```python
from build123d import *

# Parameters (mm, degrees)
SKETCH1_W                    = 73.025
SKETCH1_H                    = 177.8
BASE_FLANGE1_DEPTH           = 0.508
SKETCH2_W                    = 73.025
SKETCH2_H                    = 6.35
BOSS_EXTRUDE1_DEPTH          = 1.11125
EDGE_FLANGE1_STRIP_W         = 4.2545
EDGE_FLANGE1_STRIP_H         = 0.508
EDGE_FLANGE1_STRIP_CUT_DEPTH = 73.025
EDGE_FLANGE1_DEPTH           = 73.025


# Sheet-metal steps are written as plain solids
with BuildPart() as part:
    # Sketch1 → Base-Flange1 (new body)
    with BuildSketch(Plane(origin=(0, 0, 0), x_dir=(0, 0, -1), z_dir=(1, 0, 0))):
        with Locations((36.5125, 88.9)):
            Rectangle(SKETCH1_W, SKETCH1_H)
    extrude(amount=-BASE_FLANGE1_DEPTH)

    # Sketch2 → Boss-Extrude1 (add)
    with BuildSketch(Plane(origin=(0, 0, 0), x_dir=(0, 0, -1), z_dir=(1, 0, 0))):
        with Locations((36.5125, 174.625)):
            Rectangle(SKETCH2_W, SKETCH2_H)
    extrude(amount=BOSS_EXTRUDE1_DEPTH)

    # Edge-Flange1 strip (across the edge) → Edge-Flange1 strip cut (cut)
    with BuildSketch(Plane(origin=(-0.508, 0, -73.025), x_dir=(0, 1, 0), z_dir=(0, 0, 1))):
        with Locations((-0.508, -0.254)):
            Rectangle(EDGE_FLANGE1_STRIP_W, EDGE_FLANGE1_STRIP_H)
    extrude(amount=EDGE_FLANGE1_STRIP_CUT_DEPTH, mode=Mode.SUBTRACT)

    # Edge-Flange1 section (across the edge) → Edge-Flange1 (add)
    with BuildSketch(Plane(origin=(-0.508, 0, -73.025), x_dir=(0, 1, 0), z_dir=(0, 0, 1))):
        with BuildLine():
            Line((0, 1.11125), (0, 2.667))
            Line((0, 2.667), (0.508, 2.667))
            Line((0.508, 2.667), (0.508, 1.11125))
            ThreePointArc((0.508, 1.11125), (0.833477589, 0.325477589), (1.61925, 0))
            Line((1.61925, 0), (1.61925, -0.508))
            ThreePointArc((1.61925, -0.508), (0.474267345, -0.033732655), (0, 1.11125))
        make_face()
    extrude(amount=EDGE_FLANGE1_DEPTH)


solid = part.part
```
The model under review builds one solid part; all positions refer to its coordinate system, in mm. A direction names the side the tool comes from. Give positions to 0.01 mm unless a question says otherwise; leave off trailing zeros. Write each loop counter-clockwise with the first axis right and the second up, starting at its lowest first coordinate (ties: lowest second). Pieces come first, ordered by that corner, then holes. Notation, with made-up numbers: (89, 46.5) -> (145, 46.5) arc R14 ccw to (145, 59.5) -> close; hole circle Ø2 at (70, 52.25). An arc over 180 degrees is marked (long way). Put each result on its own line as item: value.
(1) To check wall thickness, follow probe 1 along X at (y, z) = (38, -28); probe 2 along Y at (x, z) = (0.5, -3.5); probe 3 along Y at (x, z) = (-2.3, -34). State the ranges of each line that lie inside material, in increasing order. Write a range as from..to.
Results are:
probe 1: -0.51..0
probe 2: 171.45..177.8
probe 3: 0..0.51
(2) Tool access review of faces 1 (the flat face through (-0.508, 91, -36)), 2 (the flat face through (-0.2, 95.9, -73.025)), 3 (the flat face through (0, 88, -36)): name each direction out of +Z, -Z, +X, -X, +Y, -Y from which nothing blocks a thin tool from reaching the whole face with its end or side.
Results are:
face 1: +Z, -Z, -X, +Y
face 2: -Z, +X, -X, +Y, -Y
face 3: +Z, -Z, +X, -Y
(3) We need section B-B, the plane y = 47. Give the boundary of the cut face in (x, z) (3 decimals).
Results are:
outline: (-0.508, -73.025) -> (0, -73.025) -> (0, 0) -> (-0.508, 0) -> close
(4) For pin 1 Ø3 at (y, z) = (104, -54) entering from -X; pin 2 Ø0.6 at (x, z) = (0.5, -25) entering from -Y; pin 3 Ø0.5 at (x, z) = (-2.5, -36.5) entering from +Y, all flat-tipped, find the tip position at first contact; note any pin that passes through.
Results are:
pin 1: x = -0.51
pin 2: y = 171.45
pin 3: y = 0.51
